```python
from build123d import *

# Parameters (mm, degrees)
F0_W      = 100
F0_H      = 128
F0_R      = 2.25
F0_W_2    = 68.5
F0_H_2    = 33.5
F0_W_3    = 62.5
F0_H_3    = 27.5
F1_DEPTH  = 3
F2_DEPTH  = 20
F3_DEPTH  = 4
F4_R      = 1
F5_DEPTH  = 3
F6_R      = 1
F7_DEPTH  = 3
F8_R      = 1
F9_DEPTH  = 3
F10_R     = 1
F11_DEPTH = 3


with BuildPart() as f1:
    # F0 (on Top) → F1 (new body)
    with BuildSketch(Plane.XY):
        with Locations((0, 4)):
            Rectangle(F0_W, F0_H)
        with Locations((34, -38.7)):
            Circle(F0_R, mode=Mode.SUBTRACT)
        with Locations((-44.5, 12.5)):
            Circle(F0_R, mode=Mode.SUBTRACT)
        with Locations((17, 4)):
            Circle(F0_R, mode=Mode.SUBTRACT)
        with Locations((42.5, 12.5)):
            Circle(F0_R, mode=Mode.SUBTRACT)
        with Locations((0, 45)):
            Rectangle(F0_W_2, F0_H_2, mode=Mode.SUBTRACT)
        with Locations((0, 45)):
            Rectangle(F0_W_2, F0_H_2)
        with Locations((0, 45)):
            Rectangle(F0_W_3, F0_H_3, mode=Mode.SUBTRACT)
        with Locations((-44.5, 12.5)):
            Circle(F0_R)
        with Locations((17, 4)):
            Circle(F0_R)
        with Locations((42.5, 12.5)):
            Circle(F0_R)
        with Locations((0, 45)):
            Rectangle(F0_W_3, F0_H_3)
        with Locations((34, -38.7)):
            Circle(F0_R)
    extrude(amount=-F1_DEPTH)

    # F0 (on Top) → F2 (join)
    with BuildSketch(Plane.XY):
        with Locations((-44.5, 12.5)):
            Circle(F0_R)
        with Locations((17, 4)):
            Circle(F0_R)
        with Locations((42.5, 12.5)):
            Circle(F0_R)
        with Locations((34, -38.7)):
            Circle(F0_R)
    extrude(amount=F2_DEPTH)

    # F0 (on Top) → F3 (join)
    with BuildSketch(Plane.XY):
        with Locations((0, 45)):
            Rectangle(F0_W_2, F0_H_2)
        with Locations((0, 45)):
            Rectangle(F0_W_3, F0_H_3, mode=Mode.SUBTRACT)
    extrude(amount=F3_DEPTH)

    # F4 (on face) → F5 (join)
    with BuildSketch(Plane.XY.offset(20)):
        with Locations((-44.5, 12.5)):
            Circle(F4_R)
    extrude(amount=F5_DEPTH)

    # F6 (on face) → F7 (join)
    with BuildSketch(Plane.XY.offset(20)):
        with Locations((17, 4)):
            Circle(F6_R)
    extrude(amount=F7_DEPTH)

    # F8 (on face) → F9 (join)
    with BuildSketch(Plane.XY.offset(20)):
        with Locations((42.5, 12.5)):
            Circle(F8_R)
    extrude(amount=F9_DEPTH)

    # F10 (on face) → F11 (join)
    with BuildSketch(Plane.XY.offset(20)):
        with Locations((34, -38.7)):
            Circle(F10_R)
    extrude(amount=F11_DEPTH)


solid = f1.part
```
Work out the finished part from the listing and answer in its coordinate system (mm). A direction names the side the tool comes from. Round coordinates to 2 decimals unless told otherwise and drop trailing zeros. Loops run counter-clockwise (first coordinate to the right, second up) from the corner with the lowest first, then second, coordinate; pieces in that order, holes last.
(1) For faces 5 (the flat face through (-31.25, 45, 2)), 6 (the flat face through (-1, -60, -1)), 7 (the flat face through (-3, 30, 4)), determine the directions among +Z, -Z, +X, -X, +Y, -Y from which every point of the face is accessible in a straight line to the end or side of a thin tool.
Computed values:
face 5: +Z
face 6: +Z, -Z, +X, -X, -Y
face 7: +Z, +X, -X, +Y
(2) The mould has two halves that part along X. Classify faces 1 (the cylindrical face through (19.146, 4.676, 9.86)), 2 (the flat face through (0, 61.75, 2)), 3 (the flat face through (0, 58.75, 2)), 4 (the flat face through (34.25, 45, 2)): pulls with the +X half, pulls with the -X half, needs draft (parallel to the pull), parting line crosses it, or undercut.
Computed values:
face 1: parting line crosses it
face 2: needs draft
face 3: undercut
face 4: pulls with the +X half
(3) The part is cut by section B-B, the plane z = 5.5. Give the vertices of the cut face in (x, y), and give its area (3 significant figures).
Computed values:
outline: circle Ø4.5 at (-44.5, 12.5); circle Ø4.5 at (17, 4); circle Ø4.5 at (34, -38.7); circle Ø4.5 at (42.5, 12.5)
area: 63.6 mm2
(4) Find the intervals of material crossed by L1, parallel to Y at x = -7, z = 3.5; L2, parallel to Z at x = -2, y = 33; L3, parallel to Y at x = 19, z = 8.75, in increasing order.
Computed values:
L1: y = 28.25 to 31.25, 58.75 to 61.75
L2: z = -3 to 0
L3: y = 2.97 to 5.03
(5) The part is cut by section C-C, the plane y = 18. Give the vertices of the cut face in (x, z).
Computed values:
outline: (-50, -3) - (50, -3) - (50, 0) - (-50, 0) - close
(6) Each of these flat-tipped pins is pushed along its axis until it touches: P1, Ø1.2, axis at x = 0.5, z = 2, coming from the +Y side; P2, Ø3, axis at y = 49, z = 2.5, coming from the -X side; P3, Ø4.5, axis at y = 44, z = 2.5, coming from the +X side; P4, Ø5, axis at x = -20, z = 8.5, coming from the +Y side. Where does it stop, or does it pass through?
Computed values:
P1: stops at y = 61.75
P2: stops at x = -34.25
P3: stops at x = 34.25
P4: passes through
(7) The part is cut by section A-A, the plane x = -9.5. Give the vertices of the cut face in (y, z).
Computed values:
outline: (-60, -3) - (68, -3) - (68, 0) - (61.75, 0) - (61.75, 4) - (58.75, 4) - (58.75, 0) - (31.25, 0) - (31.25, 4) - (28.25, 4) - (28.25, 0) - (-60, 0) - close
